Part print with two shaded views. Sizes in mm from the minimum x, y, z corner. A direction names the side the tool comes from. Round coordinates to 2 decimals unless told otherwise and drop trailing zeros. Loops run counter-clockwise (first coordinate to the right, second up) from the corner with the lowest first, then second, coordinate; pieces in that order, holes last. Notation, with made-up numbers: M 63.5,89 L 71.5,89 A27 cw 71.5,115 Z; hole C -32.5,7.25 d11. An arc over 180 degrees is marked long. Answer as CSV lines item,"result". Start each with the question number.
Item 1: Wall check: line 1 (Z direction, x = 12, y = 10.25); line 2 (X direction, y = 9.75, z = 29); line 3 (Y direction, x = 15.75, z = 65). Give the ranges that are in metal, low to high.
Item 2: Which spindle directions (+Z, -Z, +X, -X, +Y, -Y) get a long thin tool onto all of the face, cutting with end or side? Do the marked faces 1, 2 and 3. Say none if no direction does.
Item 3: Band-saw the part on C-C (z = 39). Give the cut face in (x, y), and give its area (3 significant figures).
Item 4: Drop flat-ended pins along their axis: pin 1 Ø5 at (y, z) = (19, 33.5) entering from +X; pin 2 Ø5 at (x, z) = (21, 27.5) entering from +Y; pin 3 Ø2 at (x, z) = (21.5, 44) entering from -Y. Give the stop position or say it passes through.
Item 5: Band-saw the part on A-A (y = 15). Give the cut face in (x, z), and give its area (3 significant figures).
Item 6: Band-saw the part on D-D (x = 25.25). Give the cut face in (y, z).
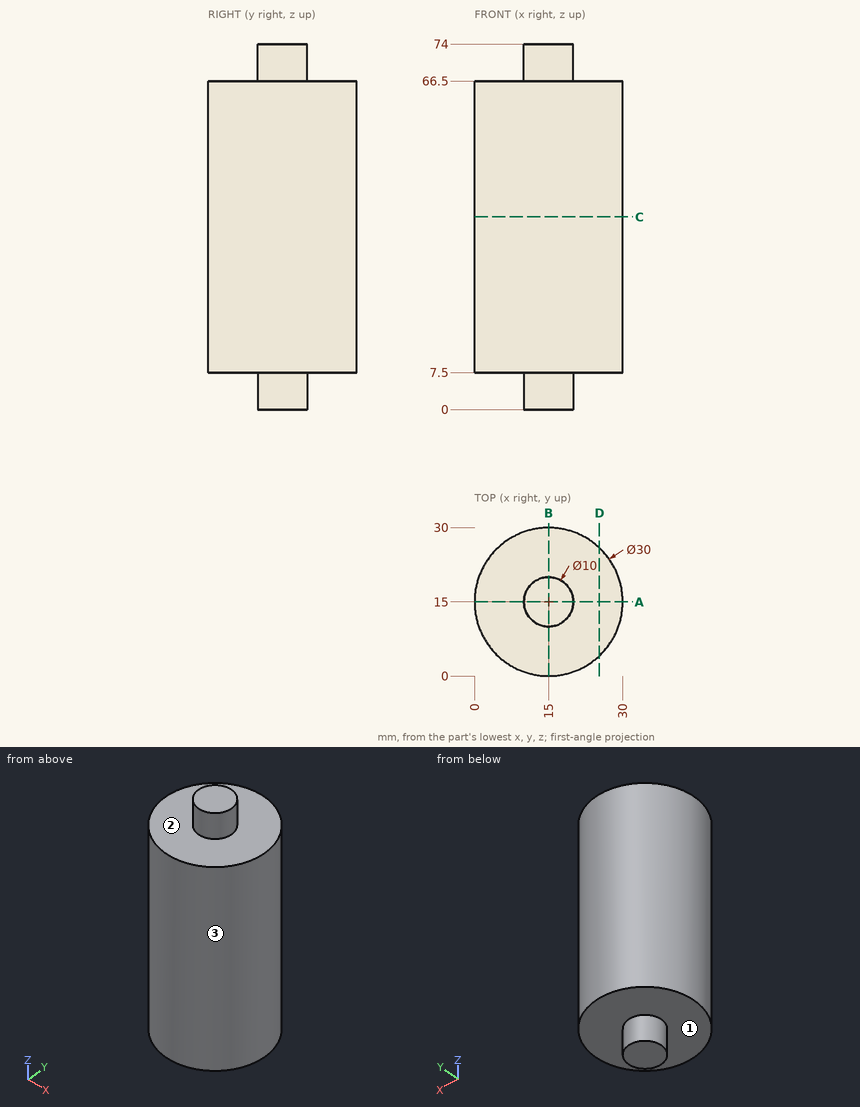
Answer block:
1,line 1,"z = 7.5 to 66.5"
1,line 2,"x = 0.95 to 29.05"
1,line 3,"y = 0.02 to 29.98"
2,face 1,"-Z"
2,face 2,"+Z"
2,face 3,"+Z, -Z"
3,outline,"C 15,15 d30"
3,area,"707 mm^2"
4,pin 1,"stops at x = 29.92"
4,pin 2,"stops at y = 29.59"
4,pin 3,"stops at y = 1.04"
5,outline,"M 0,7.5 L 10,7.5 L 10,0 L 20,0 L 20,7.5 L 30,7.5 L 30,66.5 L 20,66.5 L 20,74 L 10,74 L 10,66.5 L 0,66.5 Z"
5,area,"1,920 mm^2"
6,outline,"M 4.05,7.5 L 25.95,7.5 L 25.95,66.5 L 4.05,66.5 Z"
